from build123d import *

# Parameters (mm, degrees)
F0_R     = 2.0828
F1_DEPTH = 6.35
F0_R_2   = 3.81
F2_DEPTH = 2.7178
F4_W     = 1.27
F4_H     = 4.064
F5_DEPTH = 3.81


# Not quite as in the source:
# - a fillet or chamfer that OpenCascade refuses, or shapes differently, is made with other operations: its cross-section is extruded or revolved along the edge and cut away or added


with BuildPart() as f1:
    # F0 (on Top) → F1 (new body)
    with BuildSketch(Plane.XY):
        Circle(F0_R)
    extrude(amount=-F1_DEPTH)

    # F0 (on Top) → F2 (join)
    with BuildSketch(Plane.XY):
        Circle(F0_R_2)
        Circle(F0_R, mode=Mode.SUBTRACT)
        Circle(F0_R)
    extrude(amount=F2_DEPTH)

    # F3: fillet of radius 3.81 on 1 edges, made by hand

    # F3_s1 → F3_t2 (revolve, cut)
    with BuildSketch(Plane.XZ):
        with BuildLine():
            ThreePointArc((3.81, 0), (2.43529628, 1.9637271915), (0.1599042259, 2.7178))
            Line((0.1599042259, 2.7178), (3.81, 2.7178))
            Line((3.81, 2.7178), (3.81, 0))
        make_face()
    revolve(axis=Axis((0, 0, 2.7178), (0, 0, 1)), mode=Mode.SUBTRACT)

    # F4 (on Front) → F5 (cut, symmetric)
    with BuildSketch(Plane.XZ):
        with Locations((0, 2.7178)):
            Rectangle(F4_W, F4_H)
    extrude(amount=F5_DEPTH, both=True, mode=Mode.SUBTRACT)


solid = f1.part
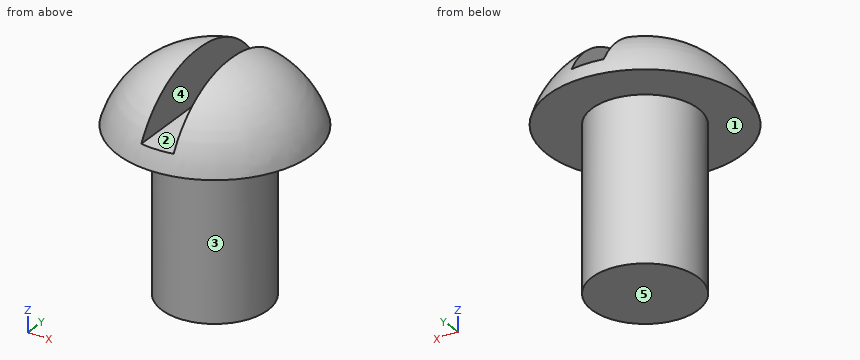
Could you check a few things on this model? Use its own coordinates, in mm. Face numbers are marked on the shaded views. A direction names the side the tool comes from. Give positions to 0.01 mm unless a question says otherwise; leave off trailing zeros. Loops run counter-clockwise (first coordinate to the right, second up) from the corner with the lowest first, then second, coordinate; pieces in that order, holes last. Notation, with made-up numbers: M 49,48 L 73,48 A4 ccw 73,54 Z; hole C 83,86.5 d4. An arc over 180 degrees is marked long. Answer as a JSON object with one key per item and string values.
Q1. If I drill on probe 1 along Z at (x, y) = (-0.25, 0.75); probe 2 along X at (y, z) = (1.75, 1) (3 decimals); probe 3 along X at (y, z) = (0.5, 0.75) (3 decimals), over which ranges is the centre line in solid material (lowest first)? Write a range as [from, to].
Values found:
{"probe 1": "z = [-6.35, 0.69]", "probe 2": "x = [-2.85, -0.635], [0.635, 2.85]", "probe 3": "x = [-3.459, -0.635], [0.635, 3.459]"}
Q2. Suppose I cut it at A-A, the plane z = -3.5. List the corners of the cut face in (x, y) for me, plus the area to 3 significant figures.
Values found:
{"outline": "C 0,0 d4.17", "area": "13.6 mm²"}
Q3. For the marked faces 1 and 2, which set-ups out of +Z, -Z, +X, -X, +Y, -Y let a thin tool reach every point of the face, with its end or its side?
Values found:
{"face 1": "-Z", "face 2": "+Z, +Y, -Y"}
Q4. For P1, Ø1, axis at x = 0.5, y = 1, coming from the +Z side; P2, Ø2, axis at y = 0, z = 2, coming from the +X side; P3, Ø3, axis at x = -2, z = 1.5, coming from the -Y side, each with a flat end and sliding along its axis, tell me the tip position at first contact or that it passes through.
Values found:
{"P1": "stops at z = 2.66", "P2": "stops at x = 3.34", "P3": "stops at y = -3.54"}
Q5. If we mould it in two halves opening along X, with no side actions, what happens to the marked faces 3, 4 and 5? For each: pulls with the +X half, pulls with the -X half, needs draft (parallel to the pull), parting line crosses it, or undercut.
Values found:
{"face 3": "parting line crosses it", "face 4": "undercut", "face 5": "needs draft"}
